Read the model definition and answer for the solid it produces. Units are mm, in the model's axes. A direction names the side the tool comes from. Coordinates: 2 decimals unless noted, no trailing zeros. Use one line per item in the form item = value. Start each with the question number.
1) Which of the six approach directions +Z, -Z, +X, -X, +Y, -Y give full straight-line access (tool end or side, diameter ignored) to faces 4 (the face through (91, 1, -3)), 5 (the face through (27.014, 19.989, -2.958))?
2) Each of these flat-tipped pins is pushed along its axis until it touches: P1, Ø3, axis at y = 20.5, z = -3, coming from the -X side; P2, Ø0.7, axis at x = 37.5, z = -2.5, coming from the +Y side (3 decimals). Where does it stop, or does it pass through?
3) The mould has two halves that part along X. Classify faces 1 (the face through (0, 10, -3)), 2 (the face through (3.45, 19.99, -2.96)), 3 (the face through (91, 11, -6)): released by +X, released by -X, zero draft, split by the parting line, or undercut.
from build123d import *

# Parameters (mm, degrees)
BLANKSKE_W              = 185
BLANKSKE_H              = 21.7
BLANK_DEPTH             = 6
TOOTHCUTSIM_DEPTH       = 187.364937689
TEETHCUTS_COUNT         = 40
TEETHCUTS_PITCH         = 4.712388975
ESQUISSE2_W             = 127.585231164
ESQUISSE2_H             = 3.375
BOSS_EXTRU_1_DEPTH      = 6
ESQUISSE3_W             = 185
ESQUISSE3_H             = 1
ENL_V_MAT_EXTRU_1_DEPTH = 6


with BuildPart() as part:
    # BlankSke → Blank (new body)
    with BuildSketch(Plane.XY):
        with Locations((92.5, 10.85)):
            Rectangle(BLANKSKE_W, BLANKSKE_H)
    extrude(amount=-BLANK_DEPTH)

    # TooCutSkeSim → ToothCutSim (cut, through all)
    with BuildSketch(Plane.XY):
        Polygon((0.654653055, 18.325), (-0.654653055, 18.325), (-1.892297439, 21.7254), (1.892297439, 21.7254), align=None)
    toothcutsim = extrude(amount=-TOOTHCUTSIM_DEPTH, mode=Mode.SUBTRACT)

    # TeethCuts: ToothCutSim ×40
    with Locations(*[(i * TEETHCUTS_PITCH, 0, 0) for i in range(1, TEETHCUTS_COUNT)]):
        add(toothcutsim, mode=Mode.SUBTRACT)

    # Esquisse2 → Boss.-Extru.1 (add)
    with BuildSketch(Plane.XY):
        with Locations((121.207384418, 20.0125)):
            Rectangle(ESQUISSE2_W, ESQUISSE2_H)
    extrude(amount=-BOSS_EXTRU_1_DEPTH)

    # Esquisse3 → Enlèv. mat.-Extru.1 (cut)
    with BuildSketch(Plane.XY):
        with Locations((92.5, 0.5)):
            Rectangle(ESQUISSE3_W, ESQUISSE3_H)
    extrude(amount=-ENL_V_MAT_EXTRU_1_DEPTH, mode=Mode.SUBTRACT)


solid = part.part
Found:
q1.face_4 = +Z, -Z, +X, -X, -Y
q1.face_5 = +Z, -Z, +Y
q2.P1 = 0.9
q2.P2 = 18.325
q3.face_1 = released by -X
q3.face_2 = undercut
q3.face_3 = zero draft
